Could you check a few things on this model? Use its own coordinates, in mm. Coordinates: 2 decimals unless noted, no trailing zeros. Write each loop counter-clockwise with the first axis right and the second up, starting at its lowest first coordinate (ties: lowest second). Pieces come first, ordered by that corner, then holes. Notation, with made-up numbers: (18.25, 22.5) - (55.25, 22.5) arc R26 cw to (55.25, 36.5) - close; hole circle Ø1 at (64, 64). An arc over 180 degrees is marked (long way). Answer as a JSON object with one key per item and string values. Group by question number.
1) Please list where these lines run through material, in increasing order: line 1 along Y through (x, z) = (0, 1.7); line 2 along X through (y, z) = (-7, 1.8); line 3 along X through (y, z) = (6, 0.2).
2) If we section it at D-D (x = -25): Write out the boundary of the cut face in (y, z), plus the area to 3 significant figures.
3) If we section it at A-A (x = 0): Write out the boundary of the cut face in (y, z).
4) If we section it at C-C (z = 1.9): Write out the boundary of the cut face in (x, y).
5) Will these pins go through, and if not, where does the flat tip stop? pin 1 Ø1.5 at (x, z) = (-11.5, 0.5) entering from -Y; pin 2 Ø0.9 at (x, z) = (1, 1.5) entering from -Y; pin 3 Ø10 at (x, y) = (62, 0) entering from -Z.
Autodesk Inventor part; units mm, degrees
ref_plane "YZ Plane" through (0, 0, 0) normal (1, 0, 0) x (0, 1, 0)
ref_plane "XZ Plane" through (0, 0, 0) normal (0, 1, 0) x (-1, 0, 0)
ref_plane "XY Plane" through (0, 0, 0) normal (0, 0, 1) x (1, 0, 0)
sketch "Sketch1" plane through (0, 0, 0) normal (0, 0, 1) x (1, 0, 0)
  circle A0 centre (0, 0) radius 78
  line L0 (28.5, 28.5) -> (-28.5, 28.5)
  line L1 (-28.5, 28.5) -> (-28.5, -28.5)
  line L2 (-28.5, -28.5) -> (28.5, -28.5)
  line L3 (28.5, -28.5) -> (28.5, 28.5)
  line L4 (28.5, 28.5) -> (-28.5, -28.5) construction
  line L5 (-28.5, 28.5) -> (28.5, -28.5) construction
  dimension "d157" = 156
  dimension "d158" = 57
  dimension "d159" = 57
extrude "Plate5" add sketch "Sketch1" along normal blind 3
sketch "Sketch7" plane through (0, 0, 0) normal (0, 0, -1) x (-1, 0, 0)
  circle A0 centre (0, 62) radius 8.5
  point P0 (0, 0)
  dimension "d160" = 17
  dimension "d161" = 62
extrude "Cut1" cut sketch "Sketch7" against normal blind 3
pattern_circular "Circular Pattern1" count 4 over 360 about axis through (0, 0, -10) along (0, 0, 1) of "Cut1"
fillet "Corner Round1" radius 6 4 edges at (-28.5, -28.5, 1.5) (28.5, -28.5, 1.5) (28.5, 28.5, 1.5) (-28.5, 28.5, 1.5)
properties part number "TZS 1757 FDS 940x50 FLANGE" material "Stainless Steel"
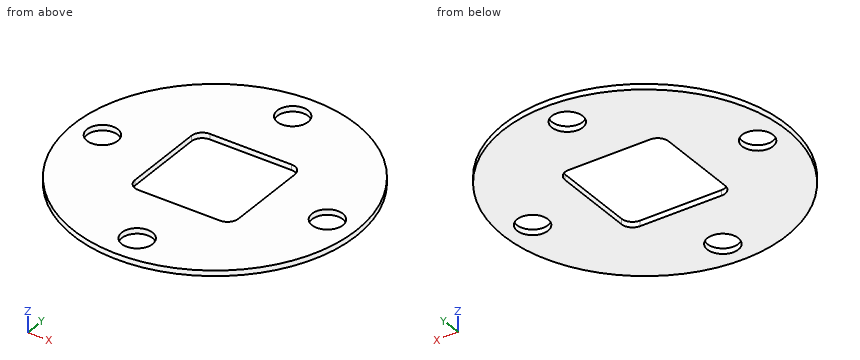
Here are the results:
{
 "1": {"line 1": "y = -78 to -70.5, -53.5 to -28.5, 28.5 to 53.5, 70.5 to 78", "line 2": "x = -77.69 to -66.82, -57.18 to -28.5, 28.5 to 57.18, 66.82 to 77.69", "line 3": "x = -77.77 to -68.02, -55.98 to -28.5, 28.5 to 55.98, 68.02 to 77.77"},
 "2": {"outline": "(-73.89, 0) - (-27.95, 0) - (-27.95, 3) - (-73.89, 3) - close; (27.95, 0) - (73.89, 0) - (73.89, 3) - (27.95, 3) - close", "area": "276 mm²"},
 "3": {"outline": "(-78, 0) - (-70.5, 0) - (-70.5, 3) - (-78, 3) - close; (-53.5, 0) - (-28.5, 0) - (-28.5, 3) - (-53.5, 3) - close; (28.5, 0) - (53.5, 0) - (53.5, 3) - (28.5, 3) - close; (70.5, 0) - (78, 0) - (78, 3) - (70.5, 3) - close"},
 "4": {"outline": "circle Ø156 at (0, 0); hole circle Ø17 at (-62, 0); hole (-28.5, -22.5) arc R6 ccw to (-22.5, -28.5) - (22.5, -28.5) arc R6 ccw to (28.5, -22.5) - (28.5, 22.5) arc R6 ccw to (22.5, 28.5) - (-22.5, 28.5) arc R6 ccw to (-28.5, 22.5) - close; hole circle Ø17 at (0, -62); hole circle Ø17 at (0, 62); hole circle Ø17 at (62, 0)"},
 "5": {"pin 1": "stops at y = -77.26", "pin 2": "stops at y = -78", "pin 3": "passes through"}
}
